from build123d import *

# Parameters (mm, degrees)
SKETCH1_W           = 20
SKETCH1_H           = 10
BOSS_EXTRUDE1_DEPTH = 2
SKETCH2_R           = 4
BOSS_EXTRUDE2_DEPTH = 6
FILLET1_R           = 1


with BuildPart() as part:
    # Sketch1 → Boss-Extrude1 (new body)
    with BuildSketch(Plane.XY):
        with Locations((0, -27.096458497)):
            Rectangle(SKETCH1_W, SKETCH1_H)
    extrude(amount=BOSS_EXTRUDE1_DEPTH)

    # Sketch2 → Boss-Extrude2 (add)
    with BuildSketch(Plane.XY.offset(2)):
        with Locations((4, -27.096458497)):
            Circle(SKETCH2_R)
    extrude(amount=BOSS_EXTRUDE2_DEPTH)

    # Fillet1
    fillet1_edges = [part.edges().sort_by_distance(p)[0] for p in [
        (-10, -22.096458497, 1),
        (10, -22.096458497, 1),
        (10, -32.096458497, 1),
        (-10, -32.096458497, 1),
    ]]
    fillet(fillet1_edges, radius=FILLET1_R)


solid = part.part
Read the model definition and answer for the solid it produces. Units are mm, in the model's axes. A direction names the side the tool comes from. Round coordinates to 2 decimals unless told otherwise and drop trailing zeros. Write each loop counter-clockwise with the first axis right and the second up, starting at its lowest first coordinate (ties: lowest second). Pieces come first, ordered by that corner, then holes. Notation, with made-up numbers: (-13.5, 58) - (0.5, 58) arc R17 ccw to (0.5, 85) - close; hole circle Ø6 at (25.25, 47.25). An arc over 180 degrees is marked (long way). Use a Markdown table: item, result.
(1) The part is cut by section C-C (z = 5.25). Write down the section's boundary in (x, y), then the cut area to 3 significant figures.
Reported:
| item | result |
|---|---|
| outline | circle Ø8 at (4, -27.1) |
| area | 50.3 mm2 |
(2) The part is cut by section B-B (y = -30). Write down the section's boundary in (x, z), then the cut area to 3 significant figures.
Reported:
| item | result |
|---|---|
| outline | (-10, 0) - (10, 0) - (10, 2) - (6.75, 2) - (6.75, 8) - (1.25, 8) - (1.25, 2) - (-10, 2) - close |
| area | 73.0 mm2 |
(3) The part is cut by section D-D (x = -6.25). Write down the section's boundary in (y, z), then the cut area to 3 significant figures.
Reported:
| item | result |
|---|---|
| outline | (-32.1, 0) - (-22.1, 0) - (-22.1, 2) - (-32.1, 2) - close |
| area | 20.0 mm2 |
(4) The part is cut by section A-A (x = 4). Write down the section's boundary in (y, z), then the cut area to 3 significant figures.
Reported:
| item | result |
|---|---|
| outline | (-32.1, 0) - (-22.1, 0) - (-22.1, 2) - (-23.1, 2) - (-23.1, 8) - (-31.1, 8) - (-31.1, 2) - (-32.1, 2) - close |
| area | 68.0 mm2 |
(5) Straight lines are drawn through the part: line 1 along Z through (x, y) = (-7.75, -29.5); line 2 along X through (y, z) = (-28.5, 7.25); line 3 along X through (y, z) = (-27.75, 5.5). For each, find the intervals that lie inside material, in ascending order. Write a range as [from, to].
Reported:
| item | result |
|---|---|
| line 1 | [0, 2] |
| line 2 | [0.25, 7.75] |
| line 3 | [0.05, 7.95] |
(6) Which of the six approach directions +Z, -Z, +X, -X, +Y, -Y give full straight-line access (tool end or side, diameter ignored) to faces 1 (the cylindrical face through (3.48, -23.13, 4.96)), 2 (the flat face through (0, -27, 0))?
Reported:
| item | result |
|---|---|
| face 1 | +Z |
| face 2 | -Z, +X, -X, +Y, -Y |
